Answer from the drawing. Dimensions are ordinates in mm from the lowest x, y and z of the part. A direction names the side the tool comes from. Give positions to 0.01 mm unless a question says otherwise; leave off trailing zeros. Loops run counter-clockwise (first coordinate to the right, second up) from the corner with the lowest first, then second, coordinate; pieces in that order, holes last. Notation, with made-up numbers: (33.25, 75.25) - (74.25, 75.25) arc R21 ccw to (74.25, 106.25) - close; hole circle Ø1 at (-7.5, 52). An arc over 180 degrees is marked (long way). One line per question, with ' | ' between items. Start each with the question number.
1. Section B-B (x = 38) is taken. Determine the outline of the cut face in (y, z), plus the area to 3 significant figures.
2. Section A-A (z = 5) is taken. Determine the outline of the cut face in (x, y), plus the area to 3 significant figures.
3. Which of the six approach directions +Z, -Z, +X, -X, +Y, -Y give full straight-line access (tool end or side, diameter ignored) to the marked faces 5 and 6?
4. Each of these flat-tipped pins is pushed along its axis until it touches: pin 1 (13.5 mm diameter, centred on x = 24, z = 12, fed in from -Y); pin 2 (12 mm diameter, centred on x = 26.5, z = 19, fed in from +Y); pin 3 (14 mm diameter, centred on x = 11.5, y = 18, fed in from +Z); pin 4 (2.5 mm diameter, centred on x = 38, z = 5, fed in from +Y). Where does it stop, or does it pass through?
5. Section D-D (y = 3.75) is taken. Determine the outline of the cut face in (x, z), plus the area to 3 significant figures.
6. Find the intervals of material crossed by line 1 (Y direction, x = 34, z = 8.5); line 2 (Z direction, x = 22, y = 4); line 3 (X direction, y = 23, z = 5.5), in increasing order.
7. For a pull along Y with two mould halves and no side action, classify the marked faces 1, 2, 3 and 4 as released by +Y, released by -Y, zero draft, split by the parting line, or undercut.
8. Section C-C (x = 13.5) is taken. Determine the outline of the cut face in (y, z).
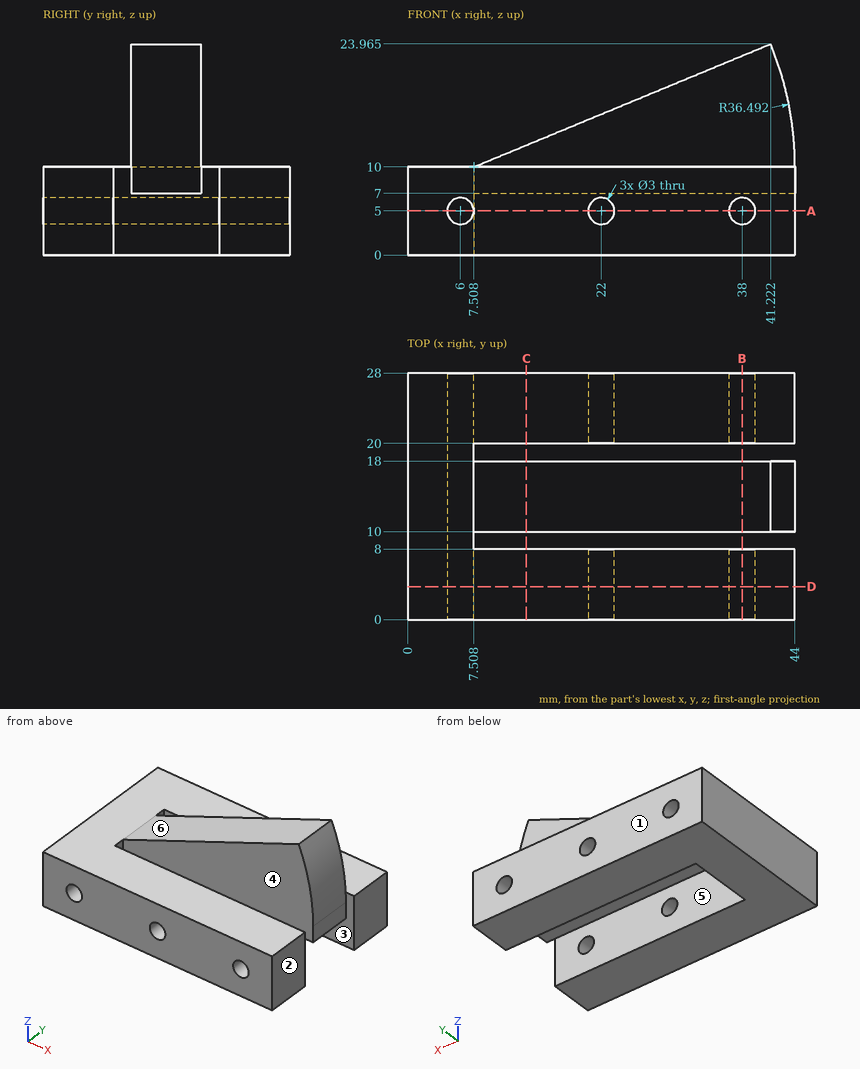
Conclusion:
1) outline: (0, 0) - (8, 0) - (8, 3.5) - (0, 3.5) - close; (0, 6.5) - (8, 6.5) - (8, 10) - (0, 10) - close; (10, 7) - (18, 7) - (18, 22.63) - (10, 22.63) - close; (20, 0) - (28, 0) - (28, 3.5) - (20, 3.5) - close; (20, 6.5) - (28, 6.5) - (28, 10) - (20, 10) - close | area: 237 mm²
2) outline: (0, 0) - (4.5, 0) - (4.5, 28) - (0, 28) - close; (7.5, 0) - (20.5, 0) - (20.5, 8) - (7.51, 8) - (7.51, 20) - (20.5, 20) - (20.5, 28) - (7.5, 28) - close; (23.5, 0) - (36.5, 0) - (36.5, 8) - (23.5, 8) - close; (23.5, 20) - (36.5, 20) - (36.5, 28) - (23.5, 28) - close; (39.5, 0) - (44, 0) - (44, 8) - (39.5, 8) - close; (39.5, 20) - (44, 20) - (44, 28) - (39.5, 28) - close | area: 614 mm²
3) face 5: +Z, -Z, +X | face 6: +Z, -X, +Y, -Y
4) pin 1: y = 0 | pin 2: y = 18 | pin 3: z = 14.55 | pin 4: through
5) outline: (0, 0) - (44, 0) - (44, 10) - (0, 10) - close; hole circle Ø3 at (6, 5); hole circle Ø3 at (22, 5); hole circle Ø3 at (38, 5) | area: 419 mm²
6) line 1: 0 to 8, 10 to 18, 20 to 28 | line 2: 0 to 3.5, 6.5 to 10 | line 3: 0 to 4.59, 7.41 to 20.59, 23.41 to 36.59, 39.41 to 44
7) face 1: released by +Y | face 2: zero draft | face 3: undercut | face 4: undercut
8) outline: (0, 0) - (8, 0) - (8, 10) - (0, 10) - close; (10, 7) - (18, 7) - (18, 12.48) - (10, 12.48) - close; (20, 0) - (28, 0) - (28, 10) - (20, 10) - close
